The listing builds one solid part. Answer for the finished solid, in the listing's coordinates (mm). A direction names the side the tool comes from. Round coordinates to 2 decimals unless told otherwise and drop trailing zeros. Loops run counter-clockwise (first coordinate to the right, second up) from the corner with the lowest first, then second, coordinate; pieces in that order, holes last. Notation, with made-up numbers: M -19.5,7.25 L 16.5,7.25 A25 cw 16.5,26.25 Z; hole C 63.25,9.5 d2. An arc over 180 degrees is marked long. Answer as a JSON object with one key per item and string values.
```python
from build123d import *

# Parameters (mm, degrees)
SKETCH1_W           = 75
SKETCH1_H           = 53
SKETCH1_R           = 1.75
BOSS_EXTRUDE8_DEPTH = 6
SKETCH6_R           = 1.6
CUT_EXTRUDE2_DEPTH  = 5


with BuildPart() as part:
    # Sketch1 → Boss-Extrude8 (new body)
    with BuildSketch(Plane(origin=(0, 0, 0), x_dir=(1, 0, 0), z_dir=(0, 1, 0))):
        with Locations((37.5, -26.5)):
            Rectangle(SKETCH1_W, SKETCH1_H)
        with Locations(Location((71.25, -6.5, 0), (0, 0, 270))):
            Circle(SKETCH1_R, mode=Mode.SUBTRACT)
        with Locations(Location((3.75, -6.5, 0), (0, 0, 270))):
            Circle(SKETCH1_R, mode=Mode.SUBTRACT)
        with Locations(Location((71.25, -46.5, 0), (0, 0, 270))):
            Circle(SKETCH1_R, mode=Mode.SUBTRACT)
        with Locations(Location((3.75, -46.5, 0), (0, 0, 270))):
            Circle(SKETCH1_R, mode=Mode.SUBTRACT)
    extrude(amount=BOSS_EXTRUDE8_DEPTH)

    # Sketch6 → Cut-Extrude2 (cut)
    with BuildSketch(Plane(origin=(0, 0, 0), x_dir=(-1, 0, 0), z_dir=(0, 0, -1))):
        with Locations((-57.5, 3)):
            Circle(SKETCH6_R)
        with Locations((-17.5, 3)):
            Circle(SKETCH6_R)
    cut_extrude2 = extrude(amount=-CUT_EXTRUDE2_DEPTH, mode=Mode.SUBTRACT)

    # Mirror1: Cut-Extrude2 across plane
    add(cut_extrude2.mirror(Plane.XY.offset(26.5)), mode=Mode.SUBTRACT)


solid = part.part
```
Item 1: The part is cut by section A-A (x = 3.75). Give the vertices of the cut face in (y, z).
Values follow:
{"outline": "M 0,0 L 6,0 L 6,4.75 L 0,4.75 Z; M 0,8.25 L 6,8.25 L 6,44.75 L 0,44.75 Z; M 0,48.25 L 6,48.25 L 6,53 L 0,53 Z"}
Item 2: Which of the six approach directions +Z, -Z, +X, -X, +Y, -Y give full straight-line access (tool end or side, diameter ignored) to faces 1 (the face through (18, 3, 5)), 2 (the face through (75, 3, 27)), 3 (the face through (18.77, 2.03, 50.54))?
Values follow:
{"face 1": "-Z", "face 2": "+Z, -Z, +X, +Y, -Y", "face 3": "+Z"}
Item 3: Straight lines are drawn through the part: line 1 (Z direction, x = 71.25, y = 3.1); line 2 (X direction, y = 3.1, z = 46.5); line 3 (X direction, y = 1.9, z = 48.5). For each, find the intervals that lie inside material, in ascending order.
Values follow:
{"line 1": "0 to 4.75, 8.25 to 44.75, 48.25 to 53", "line 2": "0 to 2, 5.5 to 69.5, 73 to 75", "line 3": "0 to 16.34, 18.66 to 56.34, 58.66 to 75"}
Item 4: Determine the mould class of faces 4 (the face through (37, 0, 26)), 5 (the face through (58, 3, 48)), 6 (the face through (3.08, 2.958, 48.117)), 7 (the face through (55.974, 3.481, 50.535)) for opening direction Y: released by +Y, released by -Y, zero draft, split by the parting line, or undercut.
Values follow:
{"face 4": "released by -Y", "face 5": "undercut", "face 6": "zero draft", "face 7": "undercut"}
Item 5: The part is cut by section C-C (y = 3). Give the vertices of the cut face in (x, z), then the cut area to 3 significant figures.
Values follow:
{"outline": "M 0,0 L 15.9,0 L 15.9,5 L 19.1,5 L 19.1,0 L 55.9,0 L 55.9,5 L 59.1,5 L 59.1,0 L 75,0 L 75,53 L 59.1,53 L 59.1,48 L 55.9,48 L 55.9,53 L 19.1,53 L 19.1,48 L 15.9,48 L 15.9,53 L 0,53 Z; hole C 3.75,6.5 d3.5; hole C 3.75,46.5 d3.5; hole C 71.25,6.5 d3.5; hole C 71.25,46.5 d3.5", "area": "3,870 mm^2"}
Item 6: A flat-ended cylindrical pin translates along its axis: P1, Ø3, axis at x = 71.25, z = 6.5, coming from the +Y side. Find the tip coordinate at first contact, or state that the pin passes through.
Values follow:
{"P1": "through"}
Item 7: The part is cut by section B-B (z = 46.5). Give the vertices of the cut face in (x, y).
Values follow:
{"outline": "M 0,0 L 2,0 L 2,6 L 0,6 Z; M 5.5,0 L 69.5,0 L 69.5,6 L 5.5,6 Z; M 73,0 L 75,0 L 75,6 L 73,6 Z"}
Item 8: The part is cut by section D-D (x = 17.5). Give the vertices of the cut face in (y, z).
Values follow:
{"outline": "M 0,0 L 1.4,0 L 1.4,5 L 4.6,5 L 4.6,0 L 6,0 L 6,53 L 4.6,53 L 4.6,48 L 1.4,48 L 1.4,53 L 0,53 Z"}
